The drawing under review shows one solid part. Ordinate dimensions are in mm from its lowest x, y, z. A direction names the side the tool comes from. Coordinates: 2 decimals unless noted, no trailing zeros. Order: outer loops, then holes, each group sorted by start corner. A loop starts at its lowest first (then second) coordinate and runs counter-clockwise, first axis right, second up. Notation, with made-up numbers: (-2, 34.5) - (51, 34.5) arc R13 ccw to (51, 56.5) - close; hole circle Ø11 at (64.25, 30.25). An arc over 180 degrees is marked (long way). Answer in a Markdown table with one row per item.
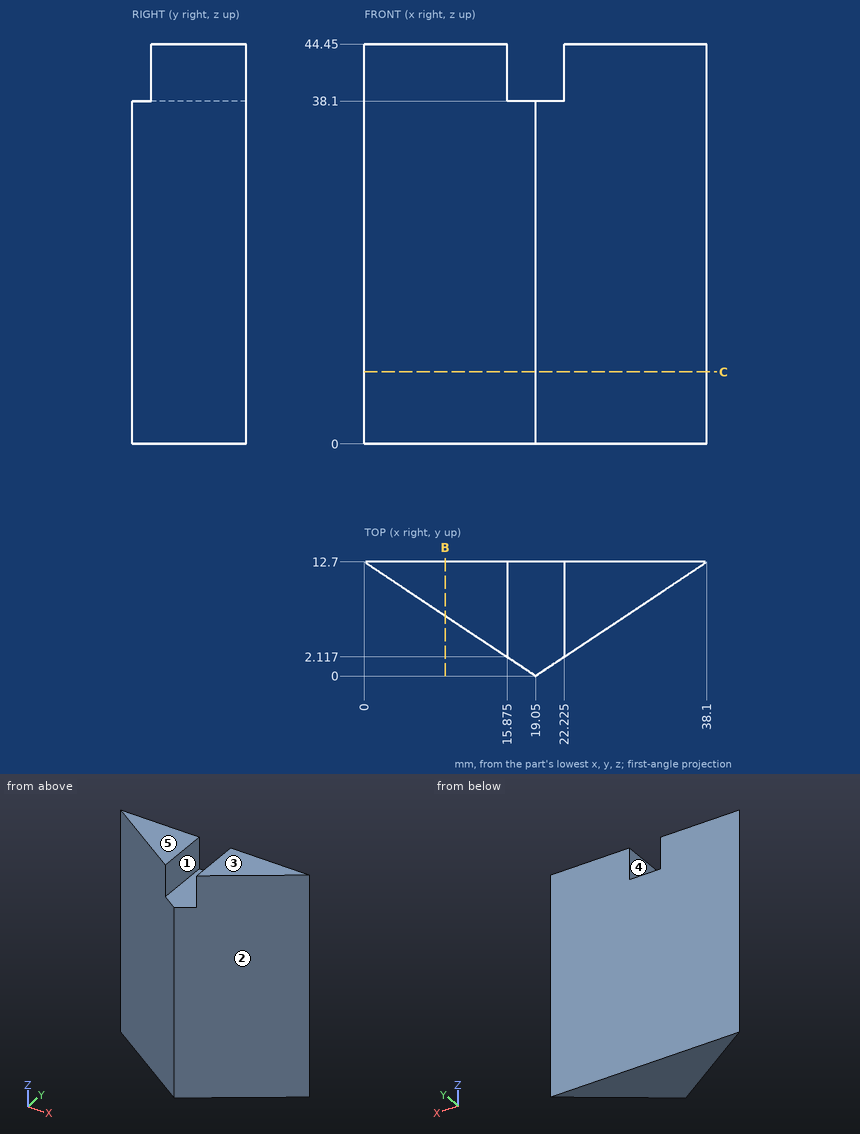
Item 1: Mouldability with a two-part tool opening along X and no side actions: class the marked faces 1, 2 and 3 as +X half, -X half, draft (parallel to the pull), parting line (faces both ways), or undercut.
Check values:
| item | result |
|---|---|
| face 1 | undercut |
| face 2 | +X half |
| face 3 | draft |
Item 2: Clearance check with flat-ended pins moving along their axes: pin 1 Ø4 at (x, z) = (23.5, 26) entering from -Y; pin 2 Ø3 at (y, z) = (4, 34.5) entering from +X; pin 3 Ø1.5 at (x, z) = (4.5, 15.5) entering from -Y. State where each tip first meets the part, or that it passes through.
Check values:
| item | result |
|---|---|
| pin 1 | y = 1.63 |
| pin 2 | x = 27.3 |
| pin 3 | y = 9.2 |
Item 3: Tool access review of the marked faces 4 and 5: name each direction out of +Z, -Z, +X, -X, +Y, -Y from which nothing blocks a thin tool from reaching the whole face with its end or side.
Check values:
| item | result |
|---|---|
| face 4 | +Z, +Y, -Y |
| face 5 | +Z, +X, -X, +Y, -Y |
Item 4: We need section B-B, the plane x = 9. Write out the cut boundary in (y, z).
Check values:
| item | result |
|---|---|
| outline | (6.7, 0) - (12.7, 0) - (12.7, 44.45) - (6.7, 44.45) - close |
Item 5: To check wall thickness, follow line 1 (Z direction, x = 19, y = 10); line 2 (Y direction, x = 33.5, z = 8.5); line 3 (Y direction, x = 24, z = 12). State the ranges of each line that lie inside material, in increasing order. Write a range as from..to.
Check values:
| item | result |
|---|---|
| line 1 | 0..38.1 |
| line 2 | 9.63..12.7 |
| line 3 | 3.3..12.7 |
Item 6: We need section C-C, the plane z = 8. Write out the cut boundary in (x, y), then the cut area to 3 significant figures.
Check values:
| item | result |
|---|---|
| outline | (0, 12.7) - (19.05, 0) - (38.1, 12.7) - close |
| area | 242 mm^2 |
